CAD build for the part. Positions are in the model's coordinates, mm. Coordinates: 2 decimals unless noted, no trailing zeros. Write each loop counter-clockwise with the first axis right and the second up, starting at its lowest first coordinate (ties: lowest second). Pieces come first, ordered by that corner, then holes. Notation, with made-up numbers: (8.25, -12.75) - (58.25, -12.75) arc R14 ccw to (58.25, 11.25) - close; hole circle Ø2 at (31, 39.25). An arc over 180 degrees is marked (long way). Answer in a Markdown table with one row per item. Add a question column.
Q1. Pin check, flat tips, straight feed: pin 1 (1.5 mm diameter, centred on y = 16, z = 30.5, fed in from +X); pin 2 (2.5 mm diameter, centred on x = -33, z = 28.5, fed in from +Y); pin 3 (3 mm diameter, centred on x = -30.5, z = 31.5, fed in from -Y). Stop position of each tip, or through.
Q2. Band-saw the part on A-A (y = 0). List the corners of the cut face in (x, z).
Q3. Drill centre lines: line 1 along Y through (x, z) = (0, 29.9); line 2 along Y through (x, z) = (15.5, 28.8); line 3 along X through (y, z) = (-27, 30.95). Where is each one in solid material? Low to high. Write a range as from..to.
Q4. Band-saw the part on C-C (z = 30.7). State how many separate pieces and enclosed holes the cut face has, and give its area (3 significant figures).
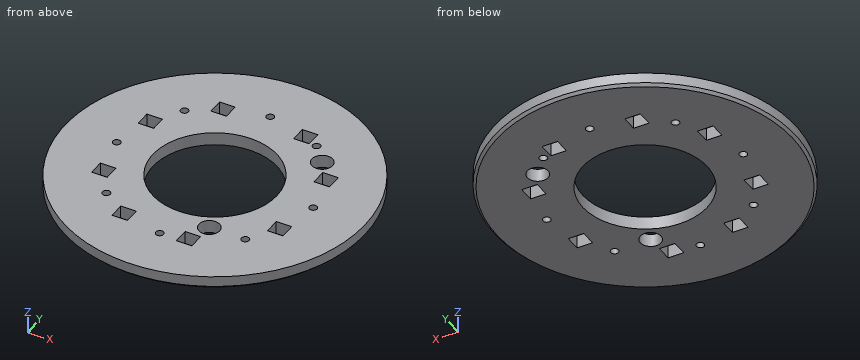
```python
from build123d import *

# Parameters (mm, degrees)
CYLINDER2136_R               = 1.5
CYLINDER2136_DEPTH           = 100
CYLINDER2139_R               = 1.5
CYLINDER2139_DEPTH           = 100
CYLINDER2139_PLACEMENT_ANGLE = 145
CYLINDER2137_R               = 1.5
CYLINDER2137_DEPTH           = 100
CYLINDER2140_R               = 1.5
CYLINDER2140_DEPTH           = 100
CYLINDER2140_PLACEMENT_ANGLE = 225
CYLINDER2141_R               = 1.5
CYLINDER2141_DEPTH           = 100
CYLINDER2142_R               = 1.5
CYLINDER2142_DEPTH           = 100
CYLINDER2142_PLACEMENT_ANGLE = 45
CYLINDER2135_R               = 1.5
CYLINDER2135_DEPTH           = 100
CYLINDER2138_R               = 1.5
CYLINDER2138_DEPTH           = 100
CYLINDER2138_PLACEMENT_ANGLE = 45
CYLINDER2113_R               = 4
CYLINDER2113_DEPTH           = 40
CYLINDER2115_R               = 4
CYLINDER2115_DEPTH           = 40
CYLINDER2118_R               = 4
CYLINDER2118_DEPTH           = 40
CYLINDER2117_R               = 4
CYLINDER2117_DEPTH           = 40
CYLINDER2112_R               = 4
CYLINDER2112_DEPTH           = 40
CYLINDER2111_R               = 4
CYLINDER2111_DEPTH           = 40
CYLINDER2116_R               = 4
CYLINDER2116_DEPTH           = 40
CYLINDER2114_R               = 4
CYLINDER2114_DEPTH           = 40
BOX1004_W                    = 6
BOX1004_H                    = 6
BOX1004_DEPTH                = 20
BOX1005_W                    = 6
BOX1005_H                    = 6
BOX1005_DEPTH                = 20
BOX1006_W                    = 6
BOX1006_H                    = 6
BOX1006_DEPTH                = 20
BOX1007_W                    = 6
BOX1007_H                    = 6
BOX1007_DEPTH                = 20
BOX1008_W                    = 6
BOX1008_H                    = 6
BOX1008_DEPTH                = 20
BOX1009_W                    = 6
BOX1009_H                    = 6
BOX1009_DEPTH                = 20
BOX1010_W                    = 6
BOX1010_H                    = 6
BOX1010_DEPTH                = 20
BOX_W                        = 6
BOX_H                        = 6
BOX_DEPTH                    = 20
TUBE088_R                    = 58
TUBE088_R_2                  = 24
TUBE088_DEPTH                = 5
CHAMFER083_SIZE              = 1


with BuildPart() as obj1:
    # Cylinder2136 → Cylinder2136 (new body)
    with BuildSketch(Plane(origin=(38, 0, 0), x_dir=(0, 1, 0), z_dir=(0, 0, 1))):
        Circle(CYLINDER2136_R)
    extrude(amount=CYLINDER2136_DEPTH)


with BuildPart() as obj2:
    # Cylinder2139 → Cylinder2139 (new body)
    with BuildSketch(Plane.XY):
        Circle(CYLINDER2139_R)
    extrude(amount=CYLINDER2139_DEPTH)


with BuildPart() as obj2_1:
    # Cylinder2139 placement: moved
    add(obj2.part.moved(Location((21.795905, 31.127778, 0))).rotate(Axis((21.795905, 31.127778, 0), (0, 0, 1)), CYLINDER2139_PLACEMENT_ANGLE))


with BuildPart() as obj3:
    # Cylinder2137 → Cylinder2137 (new body)
    with BuildSketch(Plane(origin=(0, 38, 0), x_dir=(-1, 0, 0), z_dir=(0, 0, 1))):
        Circle(CYLINDER2137_R)
    extrude(amount=CYLINDER2137_DEPTH)


with BuildPart() as obj4:
    # Cylinder2140 → Cylinder2140 (new body)
    with BuildSketch(Plane.XY):
        Circle(CYLINDER2140_R)
    extrude(amount=CYLINDER2140_DEPTH)


with BuildPart() as obj4_1:
    # Cylinder2140 placement: moved
    add(obj4.part.moved(Location((-26.870058, 26.870058, 0))).rotate(Axis((-26.870058, 26.870058, 0), (0, 0, 1)), CYLINDER2140_PLACEMENT_ANGLE))


with BuildPart() as obj5:
    # Cylinder2141 → Cylinder2141 (new body)
    with BuildSketch(Plane(origin=(-38, 0, 0), x_dir=(0, -1, 0), z_dir=(0, 0, 1))):
        Circle(CYLINDER2141_R)
    extrude(amount=CYLINDER2141_DEPTH)


with BuildPart() as obj6:
    # Cylinder2142 → Cylinder2142 (new body)
    with BuildSketch(Plane.XY):
        Circle(CYLINDER2142_R)
    extrude(amount=CYLINDER2142_DEPTH)


with BuildPart() as obj6_1:
    # Cylinder2142 placement: moved
    add(obj6.part.moved(Location((-26.870058, -26.870058, 0))).rotate(Axis((-26.870058, -26.870058, 0), (0, 0, -1)), CYLINDER2142_PLACEMENT_ANGLE))


with BuildPart() as obj7:
    # Cylinder2135 → Cylinder2135 (new body)
    with BuildSketch(Plane(origin=(0, -38, 0), x_dir=(1, 0, 0), z_dir=(0, 0, 1))):
        Circle(CYLINDER2135_R)
    extrude(amount=CYLINDER2135_DEPTH)


with BuildPart() as compound1123:
    # Cylinder2138 → Cylinder2138 (new body)
    with BuildSketch(Plane.XY):
        Circle(CYLINDER2138_R)
    extrude(amount=CYLINDER2138_DEPTH)


with BuildPart() as compound1123_1:
    # Cylinder2138 placement: moved
    add(compound1123.part.moved(Location((26.870058, -26.870058, 0))).rotate(Axis((26.870058, -26.870058, 0), (0, 0, 1)), CYLINDER2138_PLACEMENT_ANGLE))

    # Compound1123: union obj1, obj2, obj3, obj4, obj5, obj6, obj7
    add(obj1.part)
    add(obj2_1.part)
    add(obj3.part)
    add(obj4_1.part)
    add(obj5.part)
    add(obj6_1.part)
    add(obj7.part)


with BuildPart() as obj8:
    # Cylinder2113 → Cylinder2113 (new body)
    with BuildSketch(Plane(origin=(103, 12, -20), x_dir=(1, 0, 0), z_dir=(0, 0, 1))):
        Circle(CYLINDER2113_R)
    extrude(amount=CYLINDER2113_DEPTH)


with BuildPart() as obj9:
    # Cylinder2115 → Cylinder2115 (new body)
    with BuildSketch(Plane(origin=(76, 24, -18), x_dir=(1, 0, 0), z_dir=(0, 0, 1))):
        Circle(CYLINDER2115_R)
    extrude(amount=CYLINDER2115_DEPTH)


with BuildPart() as obj10:
    # Cylinder2118 → Cylinder2118 (new body)
    with BuildSketch(Plane(origin=(91, -27, -18), x_dir=(1, 0, 0), z_dir=(0, 0, 1))):
        Circle(CYLINDER2118_R)
    extrude(amount=CYLINDER2118_DEPTH)


with BuildPart() as obj11:
    # Cylinder2117 → Cylinder2117 (new body)
    with BuildSketch(Plane(origin=(13, -27, -18), x_dir=(1, 0, 0), z_dir=(0, 0, 1))):
        Circle(CYLINDER2117_R)
    extrude(amount=CYLINDER2117_DEPTH)


with BuildPart() as obj12:
    # Cylinder2112 → Cylinder2112 (new body)
    with BuildSketch(Plane(origin=(28, 24, -18), x_dir=(1, 0, 0), z_dir=(0, 0, 1))):
        Circle(CYLINDER2112_R)
    extrude(amount=CYLINDER2112_DEPTH)


with BuildPart() as obj13:
    # Cylinder2111 → Cylinder2111 (new body)
    with BuildSketch(Plane(origin=(1, -12, -18), x_dir=(1, 0, 0), z_dir=(0, 0, 1))):
        Circle(CYLINDER2111_R)
    extrude(amount=CYLINDER2111_DEPTH)


with BuildPart() as obj14:
    # Cylinder2116 → Cylinder2116 (new body)
    with BuildSketch(Plane(origin=(1, 12, -18), x_dir=(1, 0, 0), z_dir=(0, 0, 1))):
        Circle(CYLINDER2116_R)
    extrude(amount=CYLINDER2116_DEPTH)


with BuildPart() as obj15:
    # Cylinder2114 → Cylinder2114 (new body)
    with BuildSketch(Plane(origin=(103, -12, -20), x_dir=(1, 0, 0), z_dir=(0, 0, 1))):
        Circle(CYLINDER2114_R)
    extrude(amount=CYLINDER2114_DEPTH)

    # Compound1117: union obj8, obj9, obj10, obj11, obj12, obj13, obj14
    add(obj8.part)
    add(obj9.part)
    add(obj10.part)
    add(obj11.part)
    add(obj12.part)
    add(obj13.part)
    add(obj14.part)


with BuildPart() as obj15_1:
    # Compound1117 placement: moved
    add(obj15.part.moved(Location((0, 0, 20))))


with BuildPart() as krychle1004:
    # Box1004 → Box1004 (new body)
    with BuildSketch(Plane(origin=(-19, 31, 0), x_dir=(1, 0, 0), z_dir=(0, 0, 1))):
        with Locations((3, 3)):
            Rectangle(BOX1004_W, BOX1004_H)
    extrude(amount=BOX1004_DEPTH)


with BuildPart() as krychle1005:
    # Box1005 → Box1005 (new body)
    with BuildSketch(Plane(origin=(-19, -37, 0), x_dir=(1, 0, 0), z_dir=(0, 0, 1))):
        with Locations((3, 3)):
            Rectangle(BOX1005_W, BOX1005_H)
    extrude(amount=BOX1005_DEPTH)


with BuildPart() as krychle1006:
    # Box1006 → Box1006 (new body)
    with BuildSketch(Plane(origin=(7, -39, 0), x_dir=(1, 0, 0), z_dir=(0, 0, 1))):
        with Locations((3, 3)):
            Rectangle(BOX1006_W, BOX1006_H)
    extrude(amount=BOX1006_DEPTH)


with BuildPart() as krychle1007:
    # Box1007 → Box1007 (new body)
    with BuildSketch(Plane(origin=(31, 13, 0), x_dir=(1, 0, 0), z_dir=(0, 0, 1))):
        with Locations((3, 3)):
            Rectangle(BOX1007_W, BOX1007_H)
    extrude(amount=BOX1007_DEPTH)


with BuildPart() as krychle1008:
    # Box1008 → Box1008 (new body)
    with BuildSketch(Plane(origin=(31, -19, 0), x_dir=(1, 0, 0), z_dir=(0, 0, 1))):
        with Locations((3, 3)):
            Rectangle(BOX1008_W, BOX1008_H)
    extrude(amount=BOX1008_DEPTH)


with BuildPart() as krychle1009:
    # Box1009 → Box1009 (new body)
    with BuildSketch(Plane(origin=(-37, 13, 0), x_dir=(1, 0, 0), z_dir=(0, 0, 1))):
        with Locations((3, 3)):
            Rectangle(BOX1009_W, BOX1009_H)
    extrude(amount=BOX1009_DEPTH)


with BuildPart() as krychle1010:
    # Box1010 → Box1010 (new body)
    with BuildSketch(Plane(origin=(-37, -19, 0), x_dir=(1, 0, 0), z_dir=(0, 0, 1))):
        with Locations((3, 3)):
            Rectangle(BOX1010_W, BOX1010_H)
    extrude(amount=BOX1010_DEPTH)


with BuildPart() as compound1116:
    # Box → Box (new body)
    with BuildSketch(Plane(origin=(13, 31, 0), x_dir=(1, 0, 0), z_dir=(0, 0, 1))):
        with Locations((3, 3)):
            Rectangle(BOX_W, BOX_H)
    extrude(amount=BOX_DEPTH)

    # Compound1116: union Krychle1004, Krychle1005, Krychle1006, Krychle1007, Krychle1008, Krychle1009, Krychle1010
    add(krychle1004.part)
    add(krychle1005.part)
    add(krychle1006.part)
    add(krychle1007.part)
    add(krychle1008.part)
    add(krychle1009.part)
    add(krychle1010.part)


with BuildPart() as compound1116_1:
    # Compound1116 placement: moved
    add(compound1116.part.moved(Location((0, 0, 22))))


with BuildPart() as chamfer083:
    # Tube088 → Tube088 (new body)
    with BuildSketch(Plane.XY.offset(27)):
        Circle(TUBE088_R)
        Circle(TUBE088_R_2, mode=Mode.SUBTRACT)
    extrude(amount=TUBE088_DEPTH)

    # Cut705: cut Compound1116
    add(compound1116_1.part, mode=Mode.SUBTRACT)

    # Cut708: cut obj15
    add(obj15_1.part, mode=Mode.SUBTRACT)

    # Cut711: cut Compound1123
    add(compound1123_1.part, mode=Mode.SUBTRACT)

    # Chamfer083
    chamfer083_edges = [chamfer083.edges().sort_by_distance(p)[0] for p in [
        (-58, 0, 27),
    ]]
    chamfer(chamfer083_edges, length=CHAMFER083_SIZE)


solid = chamfer083.part
```
Checked values:
| question | item | result |
|---|---|---|
| 1 | pin 1 | stops at x = 55.96 |
| 1 | pin 2 | stops at y = 48.54 |
| 1 | pin 3 | stops at y = -50.23 |
| 2 | outline | (-58, 28) - (-57, 27) - (-39.5, 27) - (-39.5, 32) - (-58, 32) - close; (-36.5, 27) - (-24, 27) - (-24, 32) - (-36.5, 32) - close; (24, 27) - (36.5, 27) - (36.5, 32) - (24, 32) - close; (39.5, 27) - (57, 27) - (58, 28) - (58, 32) - (39.5, 32) - close |
| 3 | line 1 | y = -58..-39.5, -36.5..-24, 24..36.5, 39.5..58 |
| 3 | line 2 | y = -55.89..-30.12, -23.88..-18.32, 18.32..31, 37..55.89 |
| 3 | line 3 | x = -51.33..-28.36, -25.38..9, 17..25.38, 28.36..51.33 |
| 4 | separate pieces | 1 |
| 4 | enclosed holes | 19 |
| 4 | area | 8,310 mm² |
